Verification items for the finished model (mm, model axes). A direction names the side the tool comes from. Give positions to 0.01 mm unless a question says otherwise; leave off trailing zeros. Loops run counter-clockwise (first coordinate to the right, second up) from the corner with the lowest first, then second, coordinate; pieces in that order, holes last. Notation, with made-up numbers: M -16.5,77 L 40.5,77 A21 cw 40.5,82 Z; hole C 84.5,68.5 d8. An arc over 180 degrees is marked long. Use a Markdown table: item, result.
from build123d import *

# Parameters (mm, degrees)
SKETCH2_W          = 6
SKETCH2_H          = 5.3
CUT_EXTRUDE1_DEPTH = 10
SKETCH3_W          = 6
SKETCH3_H          = 3.5
CUT_EXTRUDE2_DEPTH = 8


with BuildPart() as part:
    # Sketch1 → Revolve1 (revolve)
    with BuildSketch(Plane.XY):
        Polygon((-127.75, 0), (127.75, 0), (127.75, 10), (126.25, 10), (126.25, 9.5), (124.95, 9.5), (124.95, 10), (70.75, 10), (70.75, 12.5), (47.05, 12.5), (47.05, 11.95), (45.75, 11.95), (45.75, 12.5), (30.75, 12.5), (30.75, 15), (6.75, 15), (6.75, 10), (-7.25, 10), (-7.25, 9.5), (-8.55, 9.5), (-8.55, 10), (-33.25, 10), (-33.25, 8.5), (-125.15, 8.5), (-125.15, 8.1), (-126.25, 8.1), (-126.25, 8.5), (-127.75, 8.5), align=None)
    revolve(axis=Axis((-127.75, 0, 0), (1, 0, 0)))

    # Sketch2 → Cut-Extrude1 (cut)
    with BuildSketch(Plane.ZY.offset(33.25)):
        with Locations((0, 8.15)):
            Rectangle(SKETCH2_W, SKETCH2_H)
    extrude(amount=CUT_EXTRUDE1_DEPTH, mode=Mode.SUBTRACT)

    # Sketch3 → Cut-Extrude2 (cut)
    with BuildSketch(Plane(origin=(70.75, 0, 0), x_dir=(0, 0, -1), z_dir=(1, 0, 0))):
        with Locations((0, 8.25)):
            Rectangle(SKETCH3_W, SKETCH3_H)
    extrude(amount=CUT_EXTRUDE2_DEPTH, mode=Mode.SUBTRACT)


solid = part.part
(1) Material ranges on line 1 (X direction, y = -1.5, z = -8); line 2 (X direction, y = 1, z = -10.75); line 3 (Y direction, x = 38, z = 3.5), recorded low to high.
Results below:
| item | result |
|---|---|
| line 1 | -127.75 to -126.25, -125.15 to 127.75 |
| line 2 | 6.75 to 70.75 |
| line 3 | -12 to 12 |
(2) Cross-section at B-B on x = -83. Record the cut outline in (y, z).
Results below:
| item | result |
|---|---|
| outline | C 0,0 d17 |
(3) Draft check along Z on faces 1 (the flat face through (-8.55, -9, -4)), 2 (the cylindrical face through (126.99, -2.17, -9.76)), 3 (the flat face through (75, 6.5, 0)). Enter one of: +Z half, -Z half, draft (parallel to the pull), parting line (faces both ways), or undercut.
Results below:
| item | result |
|---|---|
| face 1 | draft |
| face 2 | parting line |
| face 3 | undercut |
(4) Set-up check for faces 4 (the cylindrical face through (97.47, -2.17, -9.76)), 5 (the cylindrical face through (125.59, 4.38, -8.43)), 6 (the cylindrical face through (18.582, -14.985, 0.66)), 7 (the flat face through (127.75, 0, 0)), 8 (the flat face through (6.75, 3, -10)): record each of +Z, -Z, +X, -X, +Y, -Y from which the full face is reachable in a straight line by a thin tool's end or side.
Results below:
| item | result |
|---|---|
| face 4 | +X |
| face 5 | none |
| face 6 | +X, -X |
| face 7 | +Z, -Z, +X, +Y, -Y |
| face 8 | -X |
(5) Gauge pin test, flat ends, axial feed: P1, Ø1, axis at x = 57, z = -9, coming from the +Y side; P2, Ø2, axis at x = -39.5, y = 6.5, coming from the +Z side; P3, Ø1.8, axis at x = 76, z = 0.5, coming from the +Y side. Record the tip position at first contact, or that the pin passes through.
Results below:
| item | result |
|---|---|
| P1 | y = 9.17 |
| P2 | z = 6.48 |
| P3 | y = 6.5 |
(6) Cross-section at A-A on x = 93.5. Record the cut outline in (y, z).
Results below:
| item | result |
|---|---|
| outline | C 0,0 d20 |
